```python
from build123d import *

# Parameters (mm, degrees)
RESSALTO_EXTRUS_O1_DEPTH = 0.1
ESBO_O2_R                = 5
RESSALTO_EXTRUS_O2_DEPTH = 2
ESBO_O3_R                = 0.5
CORTE_EXTRUS_O1_DEPTH    = 10


with BuildPart() as part:
    # Esboço1 → Ressalto-extrusão1 (new body)
    with BuildSketch(Plane.XY):
        with BuildLine():
            Line((-4.617998397, 68.674835442), (5.382001603, 68.674835442))
            Line((5.382001603, 68.674835442), (5.382001603, 0.729621909))
            add(Edge.make_bspline(
                [(5.382001603, 0.729621909), (4.210394845, -19.422014325), (2.511565046, -31.255242579), (0.382001603, -31.325164558)],
                knots=[0, 0, 0, 0, 1, 1, 1, 1], degree=3))
            add(Edge.make_bspline(
                [(-4.617998397, 0.729621909), (-3.446391639, -19.422014325), (-1.747561841, -31.255242579), (0.382001603, -31.325164558)],
                knots=[0, 0, 0, 0, 1, 1, 1, 1], degree=3))
            Line((-4.617998397, 0.729621909), (-4.617998397, 68.674835442))
        make_face()
    extrude(amount=RESSALTO_EXTRUS_O1_DEPTH)

    # Esboço2 → Ressalto-extrusão2 (add)
    with BuildSketch(Plane.XY.offset(0.1)):
        with Locations(Location((0, -26.325164558, 0), (0, 0, 121.235952795))):
            Circle(ESBO_O2_R)
    extrude(amount=RESSALTO_EXTRUS_O2_DEPTH)

    # Esboço3 → Corte-extrusão1 (cut)
    with BuildSketch(Plane.XY.offset(0.1)):
        with Locations((1.682001603, 58.674835442)):
            Circle(ESBO_O3_R)
    extrude(amount=-CORTE_EXTRUS_O1_DEPTH, mode=Mode.SUBTRACT)


solid = part.part
```
Verification items for the finished model (mm, model axes). A direction names the side the tool comes from. Round coordinates to 2 decimals unless told otherwise and drop trailing zeros. Loops run counter-clockwise (first coordinate to the right, second up) from the corner with the lowest first, then second, coordinate; pieces in that order, holes last. Notation, with made-up numbers: (-36, -28.75) -> (4, -28.75) arc R28 ccw to (4, -4.75) -> close; hole circle Ø8 at (24, 42). An arc over 180 degrees is marked (long way). Answer as a JSON object with one key per item and string values.
Q1. Go/stop test with flat-tipped pins: P1, Ø1.3, axis at x = 3.5, y = -28.5, coming from the -Z side; P2, Ø2, axis at x = 2, y = 10, coming from the +Z side. Record where each tip stops, or that it passes through.
Data:
{"P1": "stops at z = 0.1", "P2": "stops at z = 0.1"}
Q2. Scan lines: line 1 (X direction, y = -22, z = 1.5); line 2 (Y direction, x = 2.75, z = 0.75); line 3 (Y direction, x = -1, z = 1.2). Record each from-to range of solid material in increasing order. Write a range as from..to.
Data:
{"line 1": "x = -2.51..2.51", "line 2": "y = -30.5..-22.15", "line 3": "y = -31.22..-21.43"}
Q3. Section check A-A (y = 53). Record the boundary of the cut face in (x, z).
Data:
{"outline": "(-4.62, 0) -> (5.38, 0) -> (5.38, 0.1) -> (-4.62, 0.1) -> close"}
Q4. Section check B-B (z = 0.65). Record the boundary of the cut face in (x, y), then the cut area to 3 significant figures.
Data:
{"outline": "circle Ø10 at (0, -26.33)", "area": "78.5 mm2"}
Q5. Access from +Z, -Z, +X, -X, +Y, -Y to the whole of each face (thin tool, end or side, straight path). Record for faces 1 (the flat face through (3, -27, 0.1)), 2 (the flat face through (0, -26, 2.1)), 3 (the cylindrical face through (2.4, -30.71, 1.09)).
Data:
{"face 1": "-Z, +X, -Y", "face 2": "+Z, +X, -X, +Y, -Y", "face 3": "+Z"}
